Autodesk Inventor part; units mm, degrees
ref_plane "YZ Plane" through (0, 0, 0) normal (1, 0, 0) x (0, 1, 0)
ref_plane "XZ Plane" through (0, 0, 0) normal (0, 1, 0) x (-1, 0, 0)
sketch "Sketch1" plane through (0, 0, 0) normal (0, 0, 1) x (1, 0, 0)
  line L0 (0, 3.937) -> (0, 34.925)
  line L1 (0, 34.925) -> (3.175, 34.925)
  line L2 (3.175, 34.925) -> (3.175, 3.175)
  line L3 (3.175, 3.175) -> (81.407, 3.175)
  line L4 (81.407, 3.175) -> (81.407, 53.975)
  line L5 (81.407, 53.975) -> (84.582, 53.975)
  line L6 (84.582, 53.975) -> (84.582, 3.937)
  line L7 (80.645, 0) -> (3.937, 0)
  arc A0 (80.645, 0) -> (84.582, 3.937) centre (80.645, 3.937) ccw
  arc A1 (0, 3.937) -> (3.937, 0) centre (3.937, 3.937) ccw
  point P0 (0, 0)
  dimension "d0" = 34.925
  dimension "d1" = 3.175
  dimension "d2" = 31.75
  dimension "d3" = 78.232
  dimension "d4" = 50.8
  dimension "d5" = 3.175
  dimension "d6" = 3.937
  dimension "d7" = 3.937
extrude "Extrusion1" add sketch "Sketch1" along normal mid plane 622.3
properties part number "2020 End Plate"
Design review of the part built by this model. Coordinates are the model's own, in mm. A direction names the side the tool comes from. Give positions to 0.01 mm unless a question says otherwise; leave off trailing zeros. Write each loop counter-clockwise with the first axis right and the second up, starting at its lowest first coordinate (ties: lowest second). Pieces come first, ordered by that corner, then holes. Notation, with made-up numbers: (62.5, -38) - (67.5, -38) arc R31 cw to (67.5, -5) - close; hole circle Ø3 at (50, 39.25). An arc over 180 degrees is marked (long way). Return JSON: item names as keys, results as strings. Group by question number.
(1) To check wall thickness, follow probe 1 along X at (y, z) = (16, 40) (3 decimals); probe 2 along Y at (x, z) = (37, 139) (3 decimals); probe 3 along X at (y, z) = (41.5, 124). State the ranges of each line that lie inside material, in increasing order.
(2) Mouldability with a two-part tool opening along X and no side actions: class faces 1 (the flat face through (43, 0, -4)), 2 (the flat face through (84.582, 29, -4)), 3 (the flat face through (3.175, 19, -4)), 4 (the flat face through (0, 19, -4)) as +X half, -X half, draft (parallel to the pull), parting line (faces both ways), or undercut.
(3) We need section A-A, the plane y = 22.5. Give the boundary of the cut face in (x, z) (3 decimals), then the cut area to 3 significant figures.
(4) We need section C-C, the plane x = 48. Give the boundary of the cut face in (y, z) (3 decimals), then the cut area to 3 significant figures.
(5) Machinability: for faces 5 (the flat face through (42, 3.175, -4)), 6 (the flat face through (45, 3, 311.15)), which of the approach directions +Z, -Z, +X, -X, +Y, -Y give a long, thin tool a straight path to every point of the face, cutting with its end or side? Answer none if there is none.
(6) Insertion check: pin 1 (1.5 mm diameter, centred on x = 18, z = 222, fed in from +Y) (3 decimals); pin 2 (1.6 mm diameter, centred on x = 1, z = -112, fed in from +Y) (3 decimals). Each pin has a flat end and moves straight along its axis. Give the tip position at first contact, or say it passes through.
(7) We need section D-D, the plane y = 48. Give the boundary of the cut face in (x, z), then the cut area to 3 significant figures.
(8) We need section B-B, the plane z = 265. Give the boundary of the cut face in (x, y) (3 decimals), then the cut area to 3 significant figures.
Reported:
{
 "1": {"probe 1": "x = 0 to 3.175, 81.407 to 84.582", "probe 2": "y = 0 to 3.175", "probe 3": "x = 81.41 to 84.58"},
 "2": {"face 1": "draft", "face 2": "+X half", "face 3": "undercut", "face 4": "-X half"},
 "3": {"outline": "(0, -311.15) - (3.175, -311.15) - (3.175, 311.15) - (0, 311.15) - close; (81.407, -311.15) - (84.582, -311.15) - (84.582, 311.15) - (81.407, 311.15) - close", "area": "3,950 mm2"},
 "4": {"outline": "(0, -311.15) - (3.175, -311.15) - (3.175, 311.15) - (0, 311.15) - close", "area": "1,980 mm2"},
 "5": {"face 5": "+Z, -Z, +Y", "face 6": "+Z, +X, -X, +Y, -Y"},
 "6": {"pin 1": "stops at y = 3.175", "pin 2": "stops at y = 34.925"},
 "7": {"outline": "(81.41, -311.15) - (84.58, -311.15) - (84.58, 311.15) - (81.41, 311.15) - close", "area": "1,980 mm2"},
 "8": {"outline": "(0, 3.937) arc R3.937 ccw to (3.937, 0) - (80.645, 0) arc R3.937 ccw to (84.582, 3.937) - (84.582, 53.975) - (81.407, 53.975) - (81.407, 3.175) - (3.175, 3.175) - (3.175, 34.925) - (0, 34.925) - close", "area": "524 mm2"}
}
